```python
from build123d import *

# Parameters (mm, degrees)
SKETCH1_W                 = 60
SKETCH1_H                 = 60
BOSS_EXTRUDE1_DEPTH       = 10
BOSS_EXTRUDE2_DEPTH       = 127
SKETCH3_W                 = 54
SKETCH3_H                 = 54
CUT_EXTRUDE1_DEPTH        = 4
SKETCH4_W                 = 26.5
SKETCH4_H                 = 4
SKETCH5_W                 = 26.5
SKETCH5_H                 = 40.4
M42_CLEARANCE_HOLE1_D     = 47
M42_CLEARANCE_HOLE1_DEPTH = 40.8
M42_CLEARANCE_HOLE2_D     = 47


with BuildPart() as part:
    # Sketch1 → Boss-Extrude1 (new body)
    with BuildSketch(Plane.XZ.offset(-47)):
        with Locations((0, -48.345395625)):
            Rectangle(SKETCH1_W, SKETCH1_H)
    extrude(amount=-BOSS_EXTRUDE1_DEPTH)

    # Sketch2 → Boss-Extrude2 (add)
    with BuildSketch(Plane.XZ.offset(-47)):
        with BuildLine():
            Line((11.939490511, -72.345395625), (30, -72.345395625))
            Line((30, -72.345395625), (30, -78.345395625))
            Line((30, -78.345395625), (-30, -78.345395625))
            Line((-30, -78.345395625), (-30, -72.345395625))
            Line((-30, -72.345395625), (-11.939490511, -72.345395625))
            ThreePointArc((-11.939490511, -72.345395625), (0, -22.187446298), (11.939490511, -72.345395625))
        make_face()
    extrude(amount=BOSS_EXTRUDE2_DEPTH)

    # Sketch3 → Cut-Extrude1 (cut)
    with BuildSketch(Plane(origin=(0, 54, 0), x_dir=(1, 0, 0), z_dir=(0, 1, 0))):
        with Locations((0, 48.345395625)):
            Rectangle(SKETCH3_W, SKETCH3_H)
    extrude(amount=-CUT_EXTRUDE1_DEPTH, mode=Mode.SUBTRACT)

    # Sketch4 → Revolve1 (revolve)
    with BuildSketch(Plane(origin=(0, 0, -48.687446298), x_dir=(-1, 0, 0), z_dir=(0, 0, -1)), mode=Mode.PRIVATE) as revolve1_sk:
        with Locations((-13.25, 52)):
            Rectangle(SKETCH4_W, SKETCH4_H)
    revolve(revolve1_sk.sketch.rotate(Axis((0, 50, -48.687446298), (0, 1, 0)), 270), axis=Axis((0, 50, -48.687446298), (0, 1, 0)))

    # Sketch5 → Revolve2 (revolve)
    with BuildSketch(Plane(origin=(0, 0, 0), x_dir=(1, 0, 0), z_dir=(0, 1, 0))):
        with Locations((13.25, 20.2)):
            Rectangle(SKETCH5_W, SKETCH5_H)
    revolve(axis=Axis((0, 0, -40.4), (0, 0, 1)))

    # M42 Clearance Hole1
    with Locations(Plane.XY):
        with Locations((0, 0)):
            Hole(M42_CLEARANCE_HOLE1_D / 2, depth=M42_CLEARANCE_HOLE1_DEPTH)

    # M42 Clearance Hole2 (through all)
    with Locations(Plane(origin=(0, -80, 0), x_dir=(-1, 0, 0), z_dir=(0, -1, 0))):
        with Locations((0, 48.687446298)):
            Hole(M42_CLEARANCE_HOLE2_D / 2)


solid = part.part
```
Work out the finished part from the listing and answer in its coordinate system (mm). A direction names the side the tool comes from. Give positions to 0.01 mm unless a question says otherwise; leave off trailing zeros. Order: outer loops, then holes, each group sorted by start corner. A loop starts at its lowest first (then second) coordinate and runs counter-clockwise, first axis right, second up.
1. Each of these flat-tipped pins is pushed along its axis until it touches: P1, Ø12, axis at y = 5, z = -23, coming from the -X side; P2, Ø10, axis at y = -61, z = -29.5, coming from the -X side; P3, Ø6, axis at x = 1, y = -8, coming from the +Z side; P4, Ø1, axis at x = 8, z = -68.5, coming from the -Y side. Where does it stop, or does it pass through?
Result sheet:
P1: stops at x = -26.5
P2: stops at x = -22.38
P3: stops at z = -71.84
P4: passes through
2. Section A-A, the plane x = 0 is taken. Determine the outline of the cut face in (y, z), and give its area (3 significant figures).
Result sheet:
outline: (-80, -78.35) - (57, -78.35) - (57, -72.19) - (-80, -72.19) - close; (-80, -25.19) - (-23.5, -25.19) - (-23.5, 0) - (-26.5, 0) - (-26.5, -22.19) - (-80, -22.19) - close; (23.5, -25.19) - (57, -25.19) - (57, -18.35) - (47, -18.35) - (47, -22.19) - (26.5, -22.19) - (26.5, 0) - (23.5, 0) - close; hole (50, -75.35) - (54, -75.35) - (54, -75.19) - (50, -75.19) - close; hole (50, -22.19) - (54, -22.19) - (54, -21.35) - (50, -21.35) - close
area: 1,280 mm2
3. The mould has two halves that part along Z. Classify faces 1 (the flat face through (0, -11, -78.345)), 2 (the flat face through (-9, 47, -23)), 3 (the flat face through (-8.1, 54, -74.5)), 4 (the flat face through (-14, 57, -28)): released by +Z, released by -Z, zero draft, split by the parting line, or undercut.
Result sheet:
face 1: released by -Z
face 2: undercut
face 3: undercut
face 4: zero draft
4. Section B-B, the plane z = -29 is taken. Determine the outline of the cut face in (x, y), and give its area (3 significant figures).
Result sheet:
outline: (-30, 47) - (-17.74, 47) - (-17.74, 19.69) arc R26.5 ccw to (-17.74, -19.69) - (-17.74, -80) - (-12.83, -80) - (-12.83, -19.69) arc R23.5 cw to (-12.83, 19.69) - (-12.83, 57) - (-30, 57) - close; (12.83, -80) - (17.74, -80) - (17.74, -19.69) arc R26.5 ccw to (17.74, 19.69) - (17.74, 47) - (30, 47) - (30, 57) - (12.83, 57) - (12.83, 19.69) arc R23.5 cw to (12.83, -19.69) - close; hole (-27, 50) - (-17.74, 50) - (-17.74, 54) - (-27, 54) - close; hole (17.74, 50) - (27, 50) - (27, 54) - (17.74, 54) - close
area: 1,400 mm2
5. For faces 5 (the cylindrical face through (-24.94, -15.61, -39.73)), 6 (the flat face through (16, -18, 0)), 7 (the cylindrical face through (24.5, -10.1, -16)), determine the directions among +Z, -Z, +X, -X, +Y, -Y from which every point of the face is accessible in a straight line to the end or side of a thin tool.
Result sheet:
face 5: none
face 6: +Z, +X, -X, +Y, -Y
face 7: +Z
6. Straight lines are drawn through the part: L1, parallel to Z at x = 0, y = -38; L2, parallel to Y at x = 0, z = -23.5; L3, parallel to Y at x = 5, z = -21.5. For each, find the intervals that lie inside material, in ascending order.
Result sheet:
L1: z = -78.35 to -72.19, -25.19 to -22.19
L2: y = -80 to -23.5, 23.5 to 57
L3: y = -26.02 to -22.96, 22.96 to 26.02, 47 to 50, 54 to 57
7. Section D-D, the plane x = -13.5 is taken. Give the number of separate pieces and of enclosed holes in the cut face, and give its area (3 significant figures).
Result sheet:
separate pieces: 3
enclosed holes: 2
area: 1,900 mm2
8. Section C-C, the plane y = 0 is taken. Determine the outline of the cut face in (x, z), and give its area (3 significant figures).
Result sheet:
outline: (-30, -78.35) - (30, -78.35) - (30, -72.35) - (11.94, -72.35) arc R26.5 ccw to (25.17, -40.4) - (26.5, -40.4) - (26.5, 0) - (23.5, 0) - (23.5, -40.8) - (22.14, -40.8) arc R23.5 cw (long way) to (-22.14, -40.8) - (-23.5, -40.8) - (-23.5, 0) - (-26.5, 0) - (-26.5, -40.4) - (-25.17, -40.4) arc R26.5 ccw to (-11.94, -72.35) - (-30, -72.35) - close
area: 842 mm2
